Can you work these out from the drawing? Everything is in mm from the part's minimum corner. A direction names the side the tool comes from. Round coordinates to 2 decimals unless told otherwise and drop trailing zeros. Write each loop counter-clockwise with the first axis right and the second up, starting at its lowest first coordinate (ties: lowest second). Pieces come first, ordered by that corner, then holes. Notation, with made-up numbers: (-32.5, -9) - (-21.5, -9) arc R3 cw to (-21.5, -5) - close; hole circle Ø11 at (21, 47). An arc over 180 degrees is marked (long way). Write each question's results on one line, items separated by ' | '. Start each with the question number.
(1) Please list where these lines run through material, in increasing order: line 1 (Y direction, x = 6, z = 2.5) (3 decimals); line 2 (Y direction, x = 3.75, z = 4.3); line 3 (Y direction, x = 2.5, z = 4.5). Write a range as [from, to].
(2) Imagine slicing it at D-D on x = 8.25. Write out the boundary of the cut face in (y, z), then the cut area to 3 significant figures.
(3) Imagine slicing it at B-B on x = 3. Write out the boundary of the cut face in (y, z) (3 decimals).
(4) For P1, Ø2.5, axis at y = 38.5, z = 2.5, coming from the -X side; P2, Ø2, axis at y = 18, z = 2, coming from the +X side, each with a flat end and sliding along its axis, tell me the tip position at first contact or that it passes through.
(5) Imagine slicing it at A-A on z = 2.5. State how many separate pieces and enclosed holes the cut face has, then the cut area to 3 significant figures.
(6) Thinking about a two-plate mould opening in Y: for the marked faces 1, 2 and 3, which applies, +Y half, -Y half, draft (parallel to the pull), parting line (faces both ways), or undercut?
(7) On a 3-axis mill with a long thin cutter (end or side, diameter ignored), from which of +Z, -Z, +X, -X, +Y, -Y can I reach the whole of each face in a straight line? I mean the marked faces 4, 5 and 6. Say none if no direction works.
(8) Imagine slicing it at C-C on y = 8.5. Write out the boundary of the cut face in (x, z) (3 decimals).
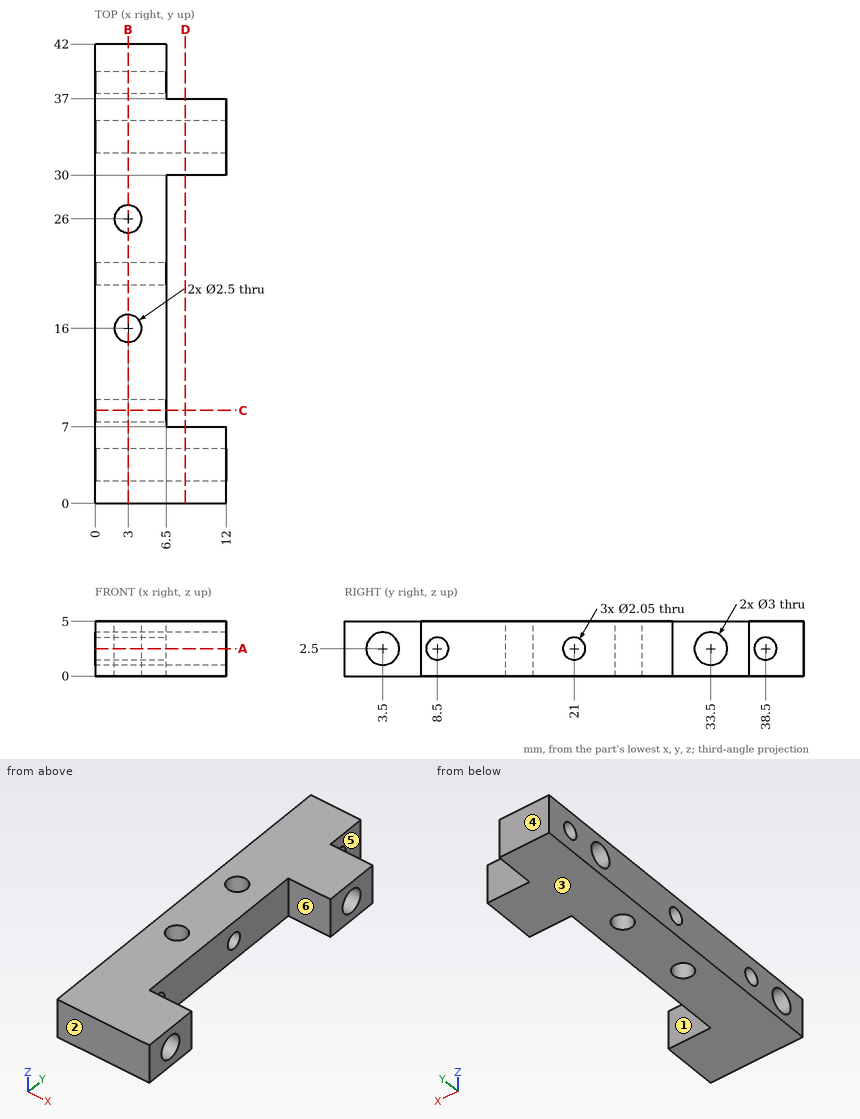
Response:
1) line 1: [0, 2], [5, 7.475], [9.525, 19.975], [22.025, 32], [35, 37.475], [39.525, 42] | line 2: [0, 15], [17, 25], [27, 42] | line 3: [0, 14.85], [17.15, 24.85], [27.15, 42]
2) outline: (0, 0) - (7, 0) - (7, 5) - (0, 5) - close; (30, 0) - (37, 0) - (37, 5) - (30, 5) - close; hole circle Ø3 at (3.5, 2.5); hole circle Ø3 at (33.5, 2.5) | area: 55.9 mm²
3) outline: (0, 0) - (14.75, 0) - (14.75, 5) - (0, 5) - close; (17.25, 0) - (24.75, 0) - (24.75, 5) - (17.25, 5) - close; (27.25, 0) - (42, 0) - (42, 5) - (27.25, 5) - close; hole circle Ø3 at (3.5, 2.5); hole circle Ø2.05 at (8.5, 2.5); hole circle Ø2.05 at (21, 2.5); hole circle Ø3 at (33.5, 2.5); hole circle Ø2.05 at (38.5, 2.5)
4) P1: x = 0 | P2: x = 6.5
5) separate pieces: 6 | enclosed holes: 2 | area: 228 mm²
6) face 1: undercut | face 2: -Y half | face 3: draft
7) face 4: +Z, -Z, +X, -X, +Y | face 5: +Z, -Z, +X, +Y | face 6: +Z, -Z, +X
8) outline: (0, 0) - (6.5, 0) - (6.5, 1.475) - (0, 1.475) - close; (0, 3.525) - (6.5, 3.525) - (6.5, 5) - (0, 5) - close
